Could you check a few things on this model? Use its own coordinates, in mm. Face numbers are marked on the shaded views. A direction names the side the tool comes from. Round coordinates to 2 decimals unless told otherwise and drop trailing zeros. Order: outer loops, then holes, each group sorted by start corner. A loop starts at its lowest first (then second) coordinate and runs counter-clockwise, first axis right, second up. Notation, with made-up numbers: M 31,58.25 L 39,58.25 A21 cw 39,68.25 Z; hole C -7,24 d9. An arc over 180 degrees is marked long. Write each question's results on one line, items separated by ' | '. Start each with the question number.
1. Suppose I cut it at C-C on z = -95. Write out the boundary of the cut face in (x, y).
2. Please list where these lines run through material, in increasing order: L1, parallel to Z at x = -3.5, y = -11.25; L2, parallel to Y at x = -9.25, z = 0; L3, parallel to X at y = -0.5, z = 94.
3. For the marked faces 1, 2 and 3, which set-ups out of +Z, -Z, +X, -X, +Y, -Y let a thin tool reach every point of the face, with its end or its side?
4. Suppose I cut it at D-D on z = -18.5. Write out the boundary of the cut face in (x, y).
5. Suppose I cut it at A-A on y = 0. Write out the boundary of the cut face in (x, z), and give its area (3 significant figures).
6. I'm going to push flat-ended pins straight in: pin 1 (1 mm diameter, centred on x = 7, y = -1, fed in from +Z); pin 2 (4 mm diameter, centred on y = -7.5, z = -8.5, fed in from -X) (3 decimals); pin 3 (8 mm diameter, centred on x = 5.5, z = -30, fed in from +Y). Where does each tip first touch, or does it pass through?
7. Suppose I cut it at B-B on x = -9.5. Write out the boundary of the cut face in (y, z), and give its area (3 significant figures).
from build123d import *

# Parameters (mm, degrees)
SKETCH3_R           = 12.5
SKETCH3_R_2         = 6.25
BOSS_EXTRUDE1_DEPTH = 60
SKETCH3_3_R         = 6.25
SKETCH3_3_R_2       = 4
BOSS_EXTRUDE2_DEPTH = 117.5
SKETCH3_4_R         = 4
BOSS_EXTRUDE3_DEPTH = 125.5
SKETCH5_R           = 7.5
CUT_EXTRUDE4_DEPTH  = 127.73890484


with BuildPart() as part:
    # Sketch3 → Boss-Extrude1 (new, symmetric)
    with BuildSketch(Plane.XY):
        Circle(SKETCH3_R)
        Circle(SKETCH3_R_2, mode=Mode.SUBTRACT)
    extrude(amount=BOSS_EXTRUDE1_DEPTH, both=True)

    # Sketch3_3 → Boss-Extrude2 (add, symmetric)
    with BuildSketch(Plane.XY):
        with Locations(Location((0, 0, 0), (0, 0, 180))):
            Circle(SKETCH3_3_R)
        with Locations(Location((0, 0, 0), (0, 0, 180))):
            Circle(SKETCH3_3_R_2, mode=Mode.SUBTRACT)
    extrude(amount=BOSS_EXTRUDE2_DEPTH, both=True)

    # Sketch3_4 → Boss-Extrude3 (add, symmetric)
    with BuildSketch(Plane.XY):
        Circle(SKETCH3_4_R)
    extrude(amount=BOSS_EXTRUDE3_DEPTH, both=True)

    # Sketch5 → Cut-Extrude4 (cut, through all)
    with BuildSketch(Plane(origin=(0, 0, 0), x_dir=(0, 0, -1), z_dir=(1, 0, 0))):
        Circle(SKETCH5_R)
    extrude(amount=-CUT_EXTRUDE4_DEPTH, mode=Mode.SUBTRACT)


solid = part.part
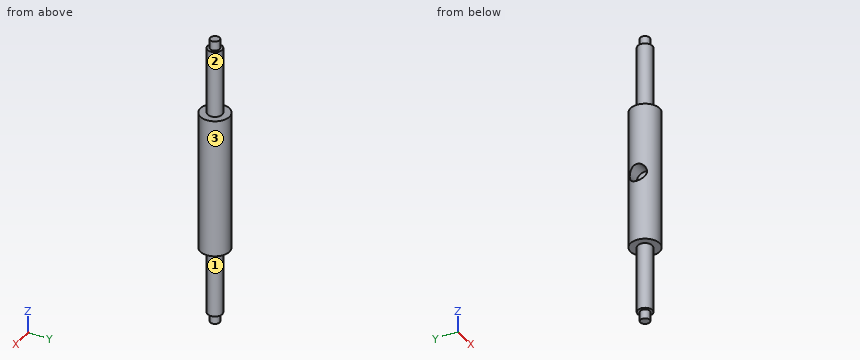
Filled sheet:
1) outline: C 0,0 d12.5
2) L1: z = -60 to 60 | L2: y = -8.41 to -7.5, 7.5 to 8.41 | L3: x = -6.23 to 6.23
3) face 1: -Z | face 2: +Z | face 3: +Z, -Z
4) outline: C 0,0 d25
5) outline: M -12.5,-60 L -6.25,-60 L -6.25,-117.5 L -4,-117.5 L -4,-125.5 L 4,-125.5 L 4,-117.5 L 6.25,-117.5 L 6.25,-60 L 12.5,-60 L 12.5,60 L 6.25,60 L 6.25,117.5 L 4,117.5 L 4,125.5 L -4,125.5 L -4,117.5 L -6.25,117.5 L -6.25,60 L -12.5,60 L -12.5,7.5 L 0,7.5 L 0,-7.5 L -12.5,-7.5 Z | area: 4,380 mm^2
6) pin 1: stops at z = 60 | pin 2: stops at x = -11.225 | pin 3: stops at y = 12.41
7) outline: M -8.12,-60 L 8.12,-60 L 8.12,60 L -8.12,60 Z; hole C 0,0 d15 | area: 1,770 mm^2
